Could you check a few things on this model? Use its own coordinates, in mm. Face numbers are marked on the shaded views. Give positions to 0.01 mm unless a question says otherwise; leave off trailing zeros. Loops run counter-clockwise (first coordinate to the right, second up) from the corner with the lowest first, then second, coordinate; pieces in that order, holes last. Notation, with made-up numbers: (41.5, -25) - (53.5, -25) arc R10 ccw to (53.5, -21) - close; hole circle Ø4 at (28, 24.5). An arc over 180 degrees is marked (long way). Use CSV: the item, a comma, the result in double quotes.
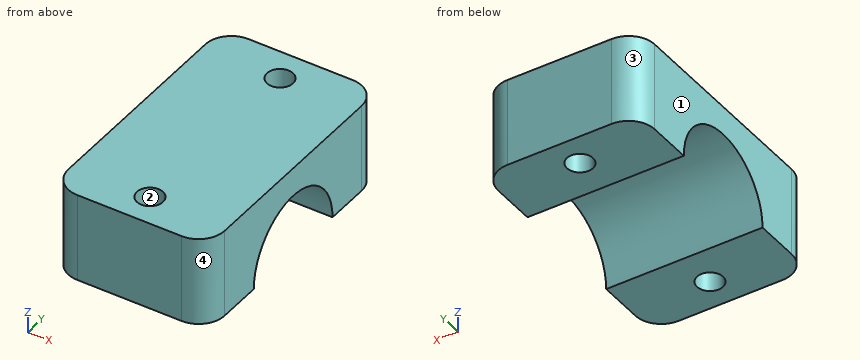
from build123d import *

# Parameters (mm, degrees)
F0_W     = 30
F0_H     = 25
F1_DEPTH = 17
F2_D     = 5
F4_DEPTH = 50
F5_R     = 5


with BuildPart() as f1:
    # F0 (on Top) → F1 (new body)
    with BuildSketch(Plane.XY):
        with Locations((0, 12.5)):
            Rectangle(F0_W, F0_H)
        with Locations((0, -12.5)):
            Rectangle(F0_W, F0_H)
    extrude(amount=F1_DEPTH)

    # F2 (through all)
    with Locations(Plane(origin=(0, 0, 0), x_dir=(1, 0, 0), z_dir=(0, 0, -1))):
        with Locations((0, 19), (0, -19)):
            Hole(F2_D / 2)

    # F3 (on face) → F4 (cut)
    with BuildSketch(Plane.YZ.offset(15)):
        with BuildLine():
            ThreePointArc((-11.5, 0), (0, -11.5), (11.5, 0))
            Line((11.5, 0), (-11.5, 0))
        make_face()
        with BuildLine():
            Line((-11.5, 0), (11.5, 0))
            ThreePointArc((11.5, 0), (0, 11.5), (-11.5, 0))
        make_face()
    extrude(amount=-F4_DEPTH, mode=Mode.SUBTRACT)

    # F5
    f5_edges = [f1.edges().sort_by_distance(p)[0] for p in [
        (15, -25, 8.5),
        (-15, -25, 8.5),
        (15, 25, 8.5),
        (-15, 25, 8.5),
    ]]
    fillet(f5_edges, radius=F5_R)


solid = f1.part
1) I need wall thicknesses on line 1 along Y through (x, z) = (0, 13.5); line 2 along X through (y, z) = (19, 13.25); line 3 along Y through (x, z) = (0, 10.25). Which ranges of each line are inside material? Lowest first, please.
Answer below:
line 1,"y = -25 to -21.5, -16.5 to 16.5, 21.5 to 25"
line 2,"x = -15 to -2.5, 2.5 to 15"
line 3,"y = -25 to -21.5, -16.5 to -5.21, 5.21 to 16.5, 21.5 to 25"
2) I'm going to push a flat-ended pin straight in: P1, Ø1.5, axis at x = -12, y = -5, coming from the -Z side. Where does the tip first touch, or does it pass through?
Answer below:
P1,"stops at z = 9.96"
3) Suppose I cut it at D-D (z = 13). Please give me the cut outline in (x, y).
Answer below:
outline,"(-15, -20) arc R5 ccw to (-10, -25) - (10, -25) arc R5 ccw to (15, -20) - (15, 20) arc R5 ccw to (10, 25) - (-10, 25) arc R5 ccw to (-15, 20) - close; hole circle Ø5 at (0, -19); hole circle Ø5 at (0, 19)"
4) Suppose I cut it at C-C (y = -19). Please give me the cut outline in (x, z).
Answer below:
outline,"(-15, 0) - (-2.5, 0) - (-2.5, 17) - (-15, 17) - close; (2.5, 0) - (15, 0) - (15, 17) - (2.5, 17) - close"
5) We'd pull the mould along Y, two halves only. Please class the marked faces 1, 2, 3 and 4: +Y half, -Y half, draft (parallel to the pull), parting line (faces both ways), or undercut.
Answer below:
face 1,"draft"
face 2,"undercut"
face 3,"+Y half"
face 4,"-Y half"
6) Suppose I cut it at A-A (x = -1.5). Please give me the cut outline in (y, z), plus the area to 3 significant figures.
Answer below:
outline,"(-25, 0) - (-21, 0) - (-21, 17) - (-25, 17) - close; (-17, 0) - (-11.5, 0) arc R11.5 cw to (11.5, 0) - (17, 0) - (17, 17) - (-17, 17) - close; (21, 0) - (25, 0) - (25, 17) - (21, 17) - close"
area,"506 mm2"
7) Suppose I cut it at B-B (z = 10.25). Please give me the cut outline in (x, y), plus the area to 3 significant figures.
Answer below:
outline,"(-15, -20) arc R5 ccw to (-10, -25) - (10, -25) arc R5 ccw to (15, -20) - (15, -5.21) - (-15, -5.21) - close; (-15, 5.21) - (15, 5.21) - (15, 20) arc R5 ccw to (10, 25) - (-10, 25) arc R5 ccw to (-15, 20) - close; hole circle Ø5 at (0, -19); hole circle Ø5 at (0, 19)"
area,"1,130 mm2"
